For this review, use the dimensioned drawing (mm, ordinates from the lowest corner) and the shaded views. Round coordinates to 2 decimals unless told otherwise and drop trailing zeros. Write each loop counter-clockwise with the first axis right and the second up, starting at its lowest first coordinate (ties: lowest second). Pieces come first, ordered by that corner, then holes. Notation, with made-up numbers: (8, -8.75) - (54, -8.75) arc R10 cw to (54, -3.75) - close; hole circle Ø5 at (-6, 57). An arc over 180 degrees is marked (long way). Return JSON: item names as keys, results as strings.
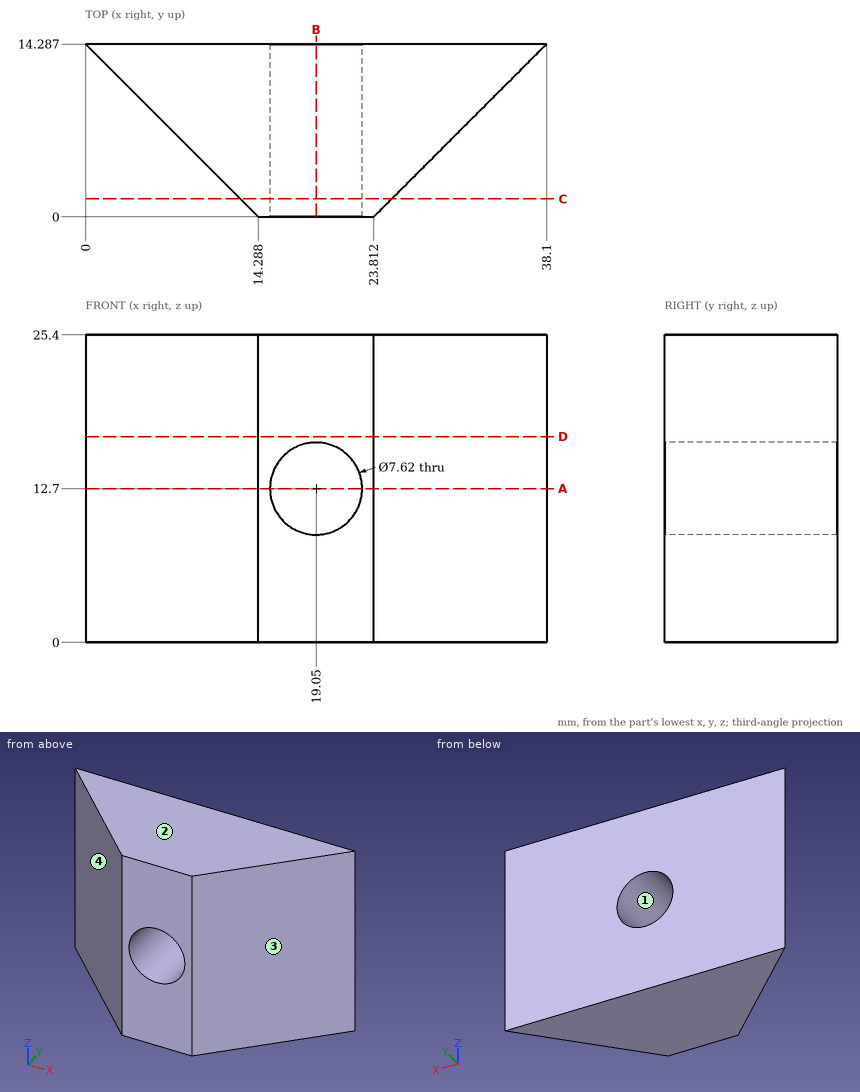
(1) Mouldability with a two-part tool opening along X and no side actions: class the marked faces 1, 2, 3 and 4 as released by +X, released by -X, zero draft, split by the parting line, or undercut.
Filled in:
{"face 1": "undercut", "face 2": "zero draft", "face 3": "released by +X", "face 4": "released by -X"}
(2) Add section C-C (y = 1.5). Write out the cut boundary in (x, z).
Filled in:
{"outline": "(12.79, 0) - (25.31, 0) - (25.31, 25.4) - (12.79, 25.4) - close; hole circle Ø7.62 at (19.05, 12.7)"}
(3) Add section D-D (z = 17). Write out the cut boundary in (x, y), plus the area to 3 significant figures.
Filled in:
{"outline": "(0, 14.29) - (14.29, 0) - (23.81, 0) - (38.1, 14.29) - close", "area": "340 mm2"}
(4) Wall thickness on line 1 (Z direction, x = 19.05, y = 6.25); line 2 (X direction, y = 12.5, z = 11.25) (1 decimal); line 3 (Y direction, x = 24, z = 23.25) (1 decimal): over which ranges is each line inside the solid? List them lowest first.
Filled in:
{"line 1": "z = 0 to 8.89, 16.51 to 25.4", "line 2": "x = 1.8 to 15.5, 22.6 to 36.3", "line 3": "y = 0.2 to 14.3"}
(5) Clearance check with flat-ended pins moving along their axes: pin 1 Ø5 at (y, z) = (2.5, 21.5) entering from -X; pin 2 Ø8 at (y, z) = (2.5, 15) entering from +X; pin 3 Ø3 at (y, z) = (2, 20.5) entering from +X. State where each tip first meets the part, or that it passes through.
Filled in:
{"pin 1": "stops at x = 9.29", "pin 2": "stops at x = 30.31", "pin 3": "stops at x = 27.31"}
(6) Add section A-A (z = 12.7). Write out the cut boundary in (x, y).
Filled in:
{"outline": "(0, 14.29) - (14.29, 0) - (15.24, 0) - (15.24, 14.29) - close; (22.86, 0) - (23.81, 0) - (38.1, 14.29) - (22.86, 14.29) - close"}
(7) Add section B-B (x = 19.05). Write out the cut boundary in (y, z).
Filled in:
{"outline": "(0, 0) - (14.29, 0) - (14.29, 8.89) - (0, 8.89) - close; (0, 16.51) - (14.29, 16.51) - (14.29, 25.4) - (0, 25.4) - close"}
